Geometry: final body of the model. Coordinates: model frame, mm. A direction names the side the tool comes from. Give positions to 0.01 mm unless a question says otherwise; leave off trailing zeros. Write each loop counter-clockwise with the first axis right and the second up, starting at its lowest first coordinate (ties: lowest second). Pieces come first, ordered by that corner, then holes. Notation, with made-up numbers: M 83.25,32 L 90.25,32 A19 cw 90.25,60 Z; hole C 63,74 d2. An arc over 180 degrees is marked long. Use a Markdown table: item, result. Add a question column.
(1) Cut plane A-A (z = 0). Output: boundary loops of the cut face in (x, y), plus the area to 3 significant figures.
(2) Material intervals for L1, parallel to X at y = 1, z = -14; L2, parallel to Y at x = 61, z = 0; L3, parallel to Z at x = 19.5, y = 0.5, sorted ascending.
(3) Pin query (flat end, axial travel): pin 1 Ø12 at (x, y) = (45.5, -10) entering from -Z; pin 2 Ø6 at (y, z) = (6, -7) entering from -X. Return the tip coordinate at first contact, or that it passes through.
(4) Cut plane B-B (y = 0). Output: boundary loops of the cut face in (x, z), plus the area to 3 significant figures.
(5) Reachability of faces 1 (the flat face through (70, -13, 4)), 2 (the flat face through (190, 0, 0)) from +Z, -Z, +X, -X, +Y, -Y: full face, straight path, thin tool, end or side. Return the list, or none.
(6) Cut plane C-C (z = -14.5). Output: boundary loops of the cut face in (x, y), plus the area to 3 significant figures.
```python
from build123d import *

# Parameters (mm, degrees)
SKETCH1_R           = 12.7
BOSS_EXTRUDE1_DEPTH = 70
SKETCH2_W           = 37.050168224
SKETCH2_H           = 34.6077549
BOSS_EXTRUDE2_DEPTH = 120


with BuildPart() as part:
    # Sketch1 → Boss-Extrude1 (new body)
    with BuildSketch(Plane.YZ):
        with Locations(Location((0, 0, 0), (0, 0, 270))):
            Circle(SKETCH1_R)
    extrude(amount=BOSS_EXTRUDE1_DEPTH)

    # Sketch2 → Boss-Extrude2 (add)
    with BuildSketch(Plane.YZ.offset(70)):
        Rectangle(SKETCH2_W, SKETCH2_H)
    extrude(amount=BOSS_EXTRUDE2_DEPTH)


solid = part.part
```
Answer list:
| question | item | result |
|---|---|---|
| 1 | outline | M 0,-12.7 L 70,-12.7 L 70,-18.53 L 190,-18.53 L 190,18.53 L 70,18.53 L 70,12.7 L 0,12.7 Z |
| 1 | area | 6,220 mm² |
| 2 | L1 | 70 to 190 |
| 2 | L2 | -12.7 to 12.7 |
| 2 | L3 | -12.69 to 12.69 |
| 3 | pin 1 | z = -12.05 |
| 3 | pin 2 | x = 0 |
| 4 | outline | M 0,-12.7 L 70,-12.7 L 70,-17.3 L 190,-17.3 L 190,17.3 L 70,17.3 L 70,12.7 L 0,12.7 Z |
| 4 | area | 5,930 mm² |
| 5 | face 1 | -X |
| 5 | face 2 | +Z, -Z, +X, +Y, -Y |
| 6 | outline | M 70,-18.53 L 190,-18.53 L 190,18.53 L 70,18.53 Z |
| 6 | area | 4,450 mm² |
